Check sheet for the drawn part. Datum: minimum x, y, z corner. Units: mm. A direction names the side the tool comes from. Round coordinates to 2 decimals unless told otherwise and drop trailing zeros. Write each loop counter-clockwise with the first axis right and the second up, starting at its lowest first coordinate (ties: lowest second). Pieces come first, ordered by that corner, then holes. Notation, with made-up numbers: (61, 1.5) - (120, 1.5) arc R34 cw to (120, 39.5) - close; hole circle Ø1 at (-34, 73). An arc over 180 degrees is marked (long way). Answer as a JSON object with one key per item and string values. Group by question number.
1) Section check A-A (z = 8). Enter the section's corners in (x, y).
2) Go/stop test with flat-tipped pins: pin 1 Ø5 at (x, z) = (41.5, 27.5) entering from -Y; pin 2 Ø3 at (y, z) = (34.5, 30.5) entering from +X; pin 3 Ø11 at (y, z) = (21, 30.5) entering from -X; pin 4 Ø5.5 at (x, y) = (7, 48) entering from +Z. Record where each tip stops, or that it passes through.
3) Mould release check, pull along X, two halves, no side actions. Record for the marked faces 4, 5, 6 and 7: +X half, -X half, draft (parallel to the pull), parting line (faces both ways), or undercut.
4) Set-up check for the marked faces 1, 2 and 3: record each of +Z, -Z, +X, -X, +Y, -Y from which the full face is reachable in a straight line by a thin tool's end or side.
5) Section check D-D (x = 25). Enter the section's corners in (y, z).
6) Section check B-B (y = 54.45). Enter the section's corners in (x, z), then the cut area to 3 significant figures.
7) Thickness scan on line 1 (X direction, y = 54, z = 8.5); line 2 (Y direction, x = 25.5, z = 23) (1 decimal); line 3 (Y direction, x = 26.5, z = 21) (1 decimal). Record the ranges inside material, lowest first.
8) Section check C-C (y = 32). Enter the section's corners in (x, z), then the cut area to 3 significant figures.
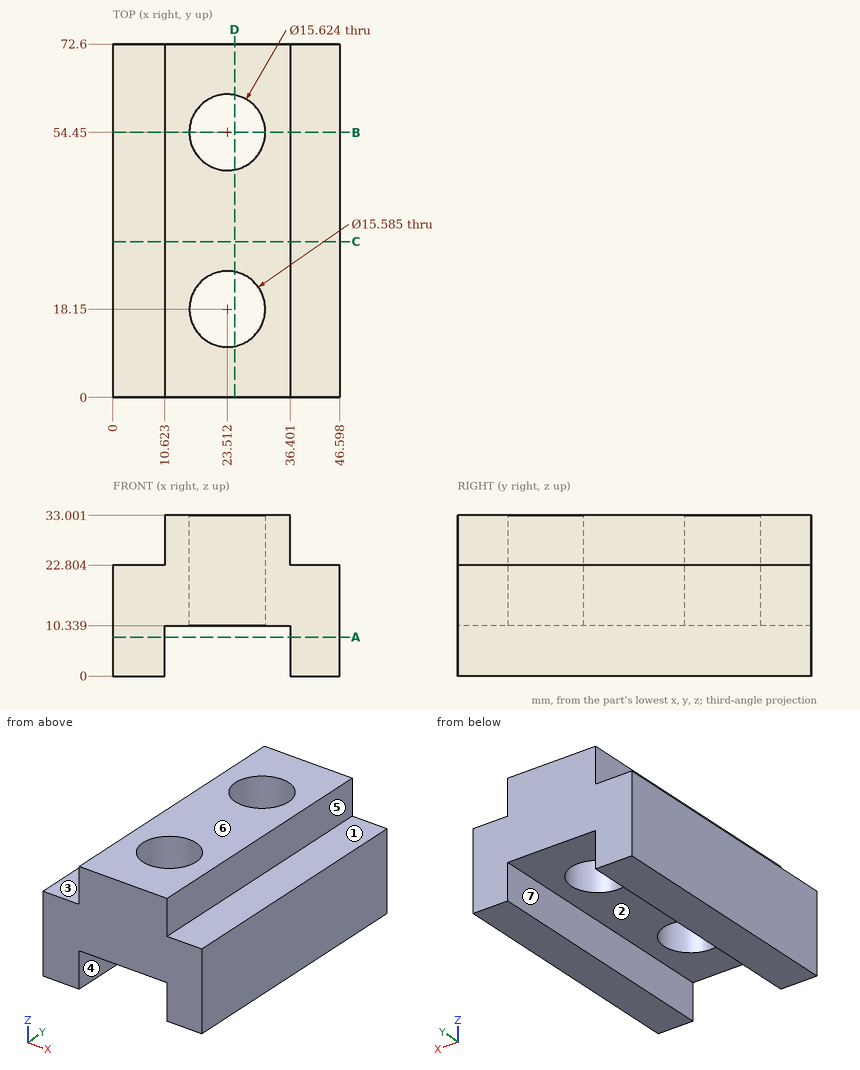
Returned:
{
 "1": {"outline": "(0, 0) - (10.62, 0) - (10.62, 72.6) - (0, 72.6) - close; (36.4, 0) - (46.6, 0) - (46.6, 72.6) - (36.4, 72.6) - close"},
 "2": {"pin 1": "through", "pin 2": "x = 36.4", "pin 3": "x = 10.62", "pin 4": "z = 22.8"},
 "3": {"face 4": "undercut", "face 5": "+X half", "face 6": "draft", "face 7": "undercut"},
 "4": {"face 1": "+Z, +X, +Y, -Y", "face 2": "-Z, +Y, -Y", "face 3": "+Z, -X, +Y, -Y"},
 "5": {"outline": "(0, 10.34) - (10.5, 10.34) - (10.5, 33) - (0, 33) - close; (25.8, 10.34) - (46.78, 10.34) - (46.78, 33) - (25.8, 33) - close; (62.12, 10.34) - (72.6, 10.34) - (72.6, 33) - (62.12, 33) - close"},
 "6": {"outline": "(0, 0) - (10.62, 0) - (10.62, 10.34) - (15.7, 10.34) - (15.7, 33) - (10.62, 33) - (10.62, 22.8) - (0, 22.8) - close; (31.32, 10.34) - (36.4, 10.34) - (36.4, 0) - (46.6, 0) - (46.6, 22.8) - (36.4, 22.8) - (36.4, 33) - (31.32, 33) - close", "area": "705 mm2"},
 "7": {"line 1": "0 to 10.62, 36.4 to 46.6", "line 2": "0 to 10.6, 25.7 to 46.9, 62 to 72.6", "line 3": "0 to 11, 25.3 to 47.2, 61.7 to 72.6"},
 "8": {"outline": "(0, 0) - (10.62, 0) - (10.62, 10.34) - (36.4, 10.34) - (36.4, 0) - (46.6, 0) - (46.6, 22.8) - (36.4, 22.8) - (36.4, 33) - (10.62, 33) - (10.62, 22.8) - (0, 22.8) - close", "area": "1,060 mm2"}
}
